from build123d import *

# Parameters (mm, degrees)
EXTRUDE_1_DEPTH = 1
EXTRUDE_2_DEPTH = 3
FILLET_1_R      = 0.3


with BuildPart() as part:
    # 草图1 → 凸台-拉伸1 (new body)
    with BuildSketch(Plane(origin=(0, 0, 0), x_dir=(0, 0, -1), z_dir=(1, 0, 0))):
        with BuildLine():
            Line((0, 2.5), (8, 2.5))
            ThreePointArc((8, 2.5), (10.5, 0), (8, -2.5))
            Line((8, -2.5), (0, -2.5))
            ThreePointArc((0, -2.5), (-2.5, 0), (0, 2.5))
        make_face()
    extrude(amount=EXTRUDE_1_DEPTH)

    # 草图2 → 凸台-拉伸2 (add)
    with BuildSketch(Plane(origin=(1, 0, 0), x_dir=(0, 0, -1), z_dir=(1, 0, 0))):
        with BuildLine():
            Line((0, 1.957135809), (8, 1.957135809))
            ThreePointArc((8, 1.957135809), (9.957135809, 0), (8, -1.957135809))
            Line((8, -1.957135809), (0, -1.957135809))
            ThreePointArc((0, -1.957135809), (-1.957135809, 0), (0, 1.957135809))
        make_face()
    extrude(amount=EXTRUDE_2_DEPTH)

    # 圆角1
    fillet_1_edges = [part.edges().sort_by_distance(p)[0] for p in [
        (1, 0, -10.5),
        (1, 2.5, -4),
        (4, 0, 1.957135809),
        (4, -1.957135809, -4),
        (4, 0, -9.957135809),
        (4, 1.957135809, -4),
        (1, 0, 2.5),
        (1, -2.5, -4),
    ]]
    fillet(fillet_1_edges, radius=FILLET_1_R)


solid = part.part
Verification items for the finished model (mm, model axes). A direction names the side the tool comes from. Give positions to 0.01 mm unless a question says otherwise; leave off trailing zeros. Order: outer loops, then holes, each group sorted by start corner. A loop starts at its lowest first (then second) coordinate and runs counter-clockwise, first axis right, second up. Notation, with made-up numbers: M 2,81.5 L 29,81.5 A9 ccw 29,88.5 Z; hole C 88,52.5 d2. An arc over 180 degrees is marked long. Use one line per item in the form item = value. Start each with the question number.
Q1. Scan lines: line 1 along Y through (x, z) = (3.1, -3); line 2 along Z through (x, y) = (1.6, 0.1); line 3 along Z through (x, y) = (2.55, -1.8). Record each from-to range of solid material in increasing order. Write a range as [from, to].
Q2. Access from +Z, -Z, +X, -X, +Y, -Y to the whole of each face (thin tool, end or side, straight path). Record for faces 1 (the cylindrical face through (2.331, 0.043, -9.957)), 2 (the flat face through (2, 1.957, -4)), 3 (the flat face through (2, -1.957, -4)).
Q3. Section check D-D (x = 0.5). Enter the section's corners in (y, z), then the cut area to 3 significant figures.
Q4. Section check C-C (x = 2.85). Enter the section's corners in (y, z), then the cut area to 3 significant figures.
Q5. Section check B-B (y = 0). Enter the section's corners in (x, z).
Q6. Go/stop test with a flat-tipped pin: pin 1 Ø0.8 at (x, z) = (2, -4) entering from +Y. Record where the tip stops, or that it passes through.
Q7. Section check A-A (z = -7). Enter the section's corners in (x, y).
Evaluation:
q1.line_1 = [-1.96, 1.96]
q1.line_2 = [-9.95, 1.95]
q1.line_3 = [-8.77, 0.77]
q2.face_1 = -Z, +X
q2.face_2 = +Z, -Z, +X, +Y
q2.face_3 = +Z, -Z, +X, -Y
q3.outline = M -2.5,-8 A2.5 ccw 2.5,-8 L 2.5,0 A2.5 ccw -2.5,0 Z
q3.area = 59.6 mm2
q4.outline = M -1.96,-8 A1.96 ccw 1.96,-8 L 1.96,0 A1.96 ccw -1.96,0 Z
q4.area = 43.3 mm2
q5.outline = M 0,-10.5 L 0.7,-10.5 A0.3 ccw 1,-10.2 L 1,-9.96 L 3.7,-9.96 A0.3 ccw 4,-9.66 L 4,1.66 A0.3 ccw 3.7,1.96 L 1,1.96 L 1,2.2 A0.3 ccw 0.7,2.5 L 0,2.5 Z
q6.pin_1 = 1.96
q7.outline = M 0,-2.5 L 0.7,-2.5 A0.3 ccw 1,-2.2 L 1,-1.96 L 3.7,-1.96 A0.3 ccw 4,-1.66 L 4,1.66 A0.3 ccw 3.7,1.96 L 1,1.96 L 1,2.2 A0.3 ccw 0.7,2.5 L 0,2.5 Z
